Geometry: final body of the model. Coordinates: model frame, mm. Give positions to 0.01 mm unless a question says otherwise; leave off trailing zeros. Write each loop counter-clockwise with the first axis right and the second up, starting at its lowest first coordinate (ties: lowest second). Pieces come first, ordered by that corner, then holes.
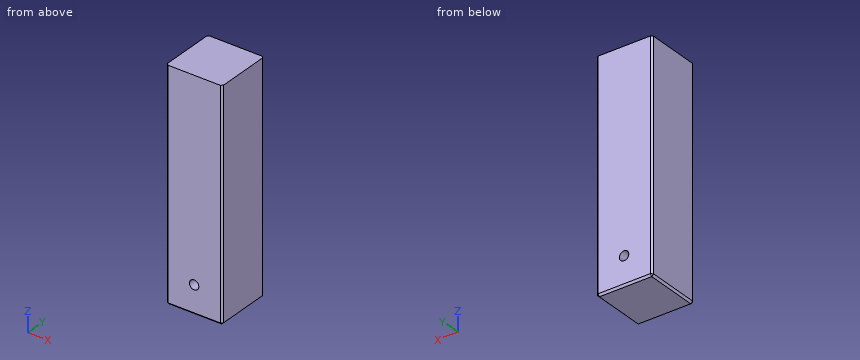
Autodesk Inventor part; units mm, degrees
ref_plane "YZ Plane" through (0, 0, 0) normal (1, 0, 0) x (0, 1, 0)
ref_plane "XZ Plane" through (0, 0, 0) normal (0, 1, 0) x (-1, 0, 0)
ref_plane "XY Plane" through (0, 0, 0) normal (0, 0, 1) x (1, 0, 0)
sketch "Skizze1" plane through (0, 0, 0) normal (0, 0, 1) x (1, 0, 0)
  line L0 (-18.741, 0) -> (23.259, 0)
  line L1 (0, -22.9262) -> (0, 19.0738)
  line L2 (-12.741, 13.0738) -> (17.259, 13.0738)
  line L3 (17.259, 13.0738) -> (17.259, -16.9262)
  line L4 (17.259, -16.9262) -> (-12.741, -16.9262)
  line L5 (-12.741, -16.9262) -> (-12.741, 13.0738)
  point P0 (0, 0)
  dimension "d0" = 30
  dimension "d1" = 30
extrude "Extrusion1" add sketch "Skizze1" along normal blind 120
sketch "Skizze2" plane through (-12.741, 13.0738, 0) normal (0, 1, 0) x (1, 0, 0)
  line L0 (0, 0) -> (0, -120)
  line L1 (30, 0) -> (0, 0)
  point P0 (12.741, 0)
  point P1 (15, -15)
  dimension "d4" = 15
  dimension "d5" = 15
hole "Bohrung1" at (2.259, 13.0738, 15) direction (0, -1, 0) diameter 5 end through all
chamfer "Fase1" distance 1 angle 45 8 edges at (17.259, 13.0738, 60) (-12.741, 13.0738, 60) (2.259, 13.0738, 0) (17.259, -1.9262, 0) (2.259, -16.9262, 0) (-12.741, -1.9262, 0) (17.259, -16.9262, 60) (-12.741, -16.9262, 60)
properties part number "Stütze mitte"
Q1. Ray query, line 1 along X through (y, z) = (-3.5, 15); line 2 along Z through (x, y) = (1, 10.5); line 3 along Z through (x, y) = (0.75, 9.5). Return the intervals inside material, ascending.
Filled sheet:
line 1: x = -12.74 to -0.24, 4.76 to 17.26
line 2: z = 0 to 12.84, 17.16 to 120
line 3: z = 0 to 13.01, 16.99 to 120
Q2. Pin query (flat end, axial travel): P1, Ø4.5, axis at x = 2.259, z = 15, coming from the -Y side. Return the tip coordinate at first contact, or that it passes through.
Filled sheet:
P1: passes through
Q3. Section A-A on z = 15. Output: boundary loops of the cut face in (x, y), plus the area to 3 significant figures.
Filled sheet:
outline: (-12.74, -15.93) - (-11.74, -16.93) - (-0.24, -16.93) - (-0.24, 13.07) - (-11.74, 13.07) - (-12.74, 12.07) - close; (4.76, -16.93) - (16.26, -16.93) - (17.26, -15.93) - (17.26, 12.07) - (16.26, 13.07) - (4.76, 13.07) - close
area: 748 mm2
